Autodesk Inventor part; units mm, degrees
ref_plane "YZ Plane" through (0, 0, 0) normal (1, 0, 0) x (0, 1, 0)
ref_plane "XZ Plane" through (0, 0, 0) normal (0, 1, 0) x (-1, 0, 0)
ref_plane "XY Plane" through (0, 0, 0) normal (0, 0, 1) x (1, 0, 0)
sketch "Sketch1" plane through (0, 0, 0) normal (0, 0, 1) x (1, 0, 0)
  circle A0 centre (0, 0) radius 9
  dimension "d0" = 18
extrude "Extrusion1" add sketch "Sketch1" along normal blind 4
sketch "Sketch3" plane through (0, 0, 4) normal (0, 0, 1) x (1, 0, 0)
  circle A0 centre (0, 0) radius 3.05
  dimension "d5" = 6.1
extrude "Extrusion3" cut sketch "Sketch3" against normal blind 2.5
sketch "Sketch4" plane through (0, 0, 0) normal (0, 0, -1) x (-1, 0, 0)
  circle A0 centre (0, 0) radius 9
  circle A1 centre (0, 0) radius 7.475
  dimension "d8" = 14.95
extrude "Extrusion4" cut sketch "Sketch4" against normal blind 3.5
sketch "Sketch5" plane through (0, 0, 4) normal (0, 0, 1) x (1, 0, 0)
  circle A0 centre (0, 0) radius 3.05
  circle A1 centre (0, 0) radius 9
extrude "Extrusion5" add sketch "Sketch5" along normal blind 1
sketch "Sketch6" plane through (0, 0, 5) normal (0, 0, 1) x (1, 0, 0)
  circle A0 centre (0, 0) radius 7.475
  circle A1 centre (0, 0) radius 9
  circle A2 centre (0, 0) radius 3.05
extrude "Extrusion6" add sketch "Sketch6" along normal blind 3 contours A0 | A1
sketch "Sketch7" plane through (0, 0, 0) normal (0, 0, -1) x (-1, 0, 0)
  circle A0 centre (0, 0) radius 7.475
extrude "Extrusion7" add sketch "Sketch7" along normal blind 3
sketch "Sketch8" plane through (0, 0, 1.5) normal (0, 0, 1) x (1, 0, 0)
  circle A0 centre (0, 0) radius 3.05
extrude "Extrusion8" add sketch "Sketch8" along normal blind 4
chamfer "Chamfer4" distance 1.5 angle 45 1 edges at (-9, 0, 8)
chamfer "Chamfer5" distance 0.3 angle 45 2 edges at (7.475, 0, -3) (-3.05, 0, 8)
properties part number "encoder_magnet_holder" material "PET Plastic"
Here's how the part is built. I have some questions about the finished solid (model axes, mm). A direction names the side the tool comes from. Give positions to 0.01 mm unless a question says otherwise; leave off trailing zeros. Loops run counter-clockwise (first coordinate to the right, second up) from the corner with the lowest first, then second, coordinate; pieces in that order, holes last. Notation, with made-up numbers: M -37.5,32 L -7.5,32 A18 ccw -7.5,49 Z; hole C 3,66 d3. An arc over 180 degrees is marked long. Put each result on its own line as item: value. Start each with the question number.
(1) I want a section at A-A on x = 0. Please give me the cut outline in (y, z) (3 decimals).
(2) I want a section at D-D on z = 0.5. Please give me the cut outline in (x, y) (3 decimals).
(3) I need wall thicknesses on line 1 along Y through (x, z) = (0, 6.15); line 2 along Y through (x, z) = (0, 2.25) (3 decimals); line 3 along Y through (x, z) = (0, 6.95). Which ranges of each line are inside material? Lowest first, please. Write a range as [from, to].
(4) I want a section at C-C on z = 6.25. Please give me the cut outline in (x, y), then the cut area to 3 significant figures.
(5) If we mould it in two halves opening along Y, with no side actions, what happens to faces 3 (the cylindrical face through (-3.047, -0.134, 6.585)), 4 (the flat face through (0, 0, 5.5)), 5 (the flat face through (0, 0, -3)), 6 (the cylindrical face through (-1.172, -8.923, 4.979))? For each: +Y half, -Y half, draft (parallel to the pull), parting line (faces both ways), or undercut.
(6) For faces 1 (the cylindrical face through (-3.45, -6.63, 0.36)), 2 (the flat face through (2, -3, 8)), which set-ups out of +Z, -Z, +X, -X, +Y, -Y let a thin tool reach every point of the face, with its end or its side?
(7) Will these pins go through, and if not, where does the flat tip stop? pin 1 Ø1.5 at (x, z) = (-1, 1) entering from -Y; pin 2 Ø1.5 at (x, y) = (-7, 6.5) entering from +Z.
Answer block:
1. outline: M -9,3.5 L -7.475,3.5 L -7.475,-2.7 L -7.175,-3 L 7.175,-3 L 7.475,-2.7 L 7.475,3.5 L 9,3.5 L 9,6.5 L 7.5,8 L 3.35,8 L 3.05,7.7 L 3.05,5.5 L -3.05,5.5 L -3.05,7.7 L -3.35,8 L -7.5,8 L -9,6.5 Z
2. outline: C 0,0 d14.95
3. line 1: [-9, -3.05], [3.05, 9]
3. line 2: [-7.475, 7.475]
3. line 3: [-8.55, -3.05], [3.05, 8.55]
4. outline: C 0,0 d18; hole C 0,0 d6.1
4. area: 225 mm^2
5. face 3: undercut
5. face 4: undercut
5. face 5: draft
5. face 6: parting line
6. face 1: -Z
6. face 2: +Z, +X, -X, +Y, -Y
7. pin 1: y = -7.47
7. pin 2: z = 6.7
